from build123d import *

# Parameters (mm, degrees)
SKETCH_1_W                   = 80
SKETCH_1_H                   = 100
EXTRUDE_1_DEPTH              = 11
SKETCH_7_W                   = 15
SKETCH_7_H                   = 30
CUT_EXTRUDE_1_DEPTH          = 16
HOLE_WIZARD_M4_1_D           = 3.3
HOLE_WIZARD_M4_1_CSINK_D     = 4.05
HOLE_WIZARD_M4_1_CSINK_ANGLE = 90
FILLET_1_R                   = 20
FILLET_2_R                   = 2
SKETCH_9_W                   = 6
SKETCH_9_H                   = 35
CUT_EXTRUDE_2_DEPTH          = 11
SKETCH_11_R                  = 3
CUT_EXTRUDE_4_DEPTH          = 15
SKETCH_15_R                  = 1.9
CUT_EXTRUDE_8_DEPTH          = 14
SKETCH_16_R                  = 4.52
CUT_EXTRUDE_9_DEPTH          = 8.5
CUT_EXTRUDE_10_DEPTH         = 8.5
CUT_EXTRUDE_11_DEPTH         = 13.5
FILLET_4_R                   = 5
FILLET_5_R                   = 2


with BuildPart() as part:
    # 草图1 → 凸台-拉伸1 (new body)
    with BuildSketch(Plane.XY):
        Rectangle(SKETCH_1_W, SKETCH_1_H)
    extrude(amount=EXTRUDE_1_DEPTH)

    # 草图7 → 切除-拉伸1 (cut)
    with BuildSketch(Plane.XY.offset(11)):
        with Locations((0, 35)):
            Rectangle(SKETCH_7_W, SKETCH_7_H)
    extrude(amount=-CUT_EXTRUDE_1_DEPTH, mode=Mode.SUBTRACT)

    # M4 螺纹孔1 (through all)
    with Locations(Plane(origin=(13.5, 24.75, 0), x_dir=(-1, 0, 0), z_dir=(0, 0, -1))):
        with Locations((0, 0), (27, 0), (41.5, -49.5), (-14.5, -49.5)):
            CounterSinkHole(HOLE_WIZARD_M4_1_D / 2, HOLE_WIZARD_M4_1_CSINK_D / 2, counter_sink_angle=HOLE_WIZARD_M4_1_CSINK_ANGLE)

    # 圆角1
    fillet_1_edges = [part.edges().sort_by_distance(p)[0] for p in [
        (-40, 50, 5.5),
        (40, 50, 5.5),
    ]]
    fillet(fillet_1_edges, radius=FILLET_1_R)

    # 圆角2
    fillet_2_edges = [part.edges().sort_by_distance(p)[0] for p in [
        (-7.5, 20, 5.5),
        (-7.5, 50, 5.5),
        (7.5, 50, 5.5),
        (7.5, 20, 5.5),
        (40, -50, 5.5),
        (-40, -50, 5.5),
    ]]
    fillet(fillet_2_edges, radius=FILLET_2_R)

    # 草图9 → 切除-拉伸2 (cut)
    with BuildSketch(Plane.XY):
        with Locations((37, 0)):
            Rectangle(SKETCH_9_W, SKETCH_9_H)
        with Locations((-37, 0)):
            Rectangle(SKETCH_9_W, SKETCH_9_H)
    extrude(amount=CUT_EXTRUDE_2_DEPTH, mode=Mode.SUBTRACT)

    # 草图11 → 切除-拉伸4 (cut)
    with BuildSketch(Plane.XY):
        with Locations((-22.273863607, 38.273863607)):
            Circle(SKETCH_11_R)
        with Locations((22.273863607, 38.273863607)):
            Circle(SKETCH_11_R)
        with Locations((22.273863607, -6.273863607)):
            Circle(SKETCH_11_R)
        with Locations((-22.273863607, -6.273863607)):
            Circle(SKETCH_11_R)
    extrude(amount=CUT_EXTRUDE_4_DEPTH, mode=Mode.SUBTRACT)

    # 草图15 → 切除-拉伸8 (cut)
    with BuildSketch(Plane.XY.offset(11)):
        with Locations((-13.5, 24.75)):
            Circle(SKETCH_15_R)
        with Locations((-28, -24.75)):
            Circle(SKETCH_15_R)
        with Locations(Location((13.5, 24.75, 0), (0, 0, 180))):
            Circle(SKETCH_15_R)
        with Locations(Location((28, -24.75, 0), (0, 0, 180))):
            Circle(SKETCH_15_R)
    extrude(amount=-CUT_EXTRUDE_8_DEPTH, mode=Mode.SUBTRACT)

    # 草图16 → 切除-拉伸9 (cut)
    with BuildSketch(Plane(origin=(0, 0, 0), x_dir=(-1, 0, 0), z_dir=(0, 0, -1))):
        with Locations((-22.273863607, 38.273863607)):
            Circle(SKETCH_16_R)
        with Locations((-22.273863607, -6.273863607)):
            Circle(SKETCH_16_R)
        with Locations(Location((22.273863607, -6.273863607, 0), (0, 0, 180))):
            Circle(SKETCH_16_R)
        with Locations(Location((22.273863607, 38.273863607, 0), (0, 0, 180))):
            Circle(SKETCH_16_R)
    extrude(amount=-CUT_EXTRUDE_9_DEPTH, mode=Mode.SUBTRACT)

    # 草图17 → 切除-拉伸10 (cut)
    with BuildSketch(Plane.XY.offset(11)):
        Polygon((-15.468764418, 21.34), (-11.531235582, 21.34), (-9.562471164, 24.75), (-11.531235582, 28.16), (-15.468764418, 28.16), (-17.437528836, 24.75), align=None)
        Polygon((-26.031235582, -28.16), (-24.062471164, -24.75), (-26.031235582, -21.34), (-29.968764418, -21.34), (-31.937528836, -24.75), (-29.968764418, -28.16), align=None)
        Polygon((29.968764418, -28.16), (26.031235582, -28.16), (24.062471164, -24.75), (26.031235582, -21.34), (29.968764418, -21.34), (31.937528836, -24.75), align=None)
        Polygon((17.437528836, 24.75), (15.468764418, 21.34), (11.531235582, 21.34), (9.562471164, 24.75), (11.531235582, 28.16), (15.468764418, 28.16), align=None)
    extrude(amount=-CUT_EXTRUDE_10_DEPTH, mode=Mode.SUBTRACT)

    # 草图18 → 切除-拉伸11 (cut)
    with BuildSketch(Plane.XY.offset(11)):
        Polygon((-52.225177231, -29.5), (-20, -29.5), (-20, -24.5), (20, -24.5), (20, -29.5), (49.13660357, -29.5), (49.13660357, -55.082609568), (-52.225177231, -55.082609568), align=None)
    extrude(amount=-CUT_EXTRUDE_11_DEPTH, mode=Mode.SUBTRACT)

    # 圆角4
    fillet_4_edges = [part.edges().sort_by_distance(p)[0] for p in [
        (40, -29.5, 5.5),
        (-40, -29.5, 5.5),
    ]]
    fillet(fillet_4_edges, radius=FILLET_4_R)

    # 圆角5
    fillet_5_edges = [part.edges().sort_by_distance(p)[0] for p in [
        (-20, -27, 0),
        (-20, -29.5, 5.5),
        (0, -24.5, 0),
        (-20, -24.5, 5.5),
        (20, -27, 0),
        (20, -24.5, 5.5),
        (20, -29.5, 5.5),
        (20, -27, 11),
        (0, -24.5, 11),
        (-20, -27, 11),
    ]]
    fillet(fillet_5_edges, radius=FILLET_5_R)


solid = part.part
Check sheet for the modelled part. Datum: model origin and axes. Units: mm. A direction names the side the tool comes from. Give positions to 0.01 mm unless a question says otherwise; leave off trailing zeros. Write each loop counter-clockwise with the first axis right and the second up, starting at its lowest first coordinate (ties: lowest second). Pieces come first, ordered by that corner, then holes. Notation, with made-up numbers: (-4.5, -11) -> (2.5, -11) arc R25 ccw to (2.5, 19) -> close; hole circle Ø8 at (-22.75, -7). An arc over 180 degrees is marked (long way). Write item = value, one per line.
Item 1: Tool access check on faces 1 (the flat face through (30.967, -26.431, 6.81)), 2 (the flat face through (7.5, 35, 6)), 3 (the flat face through (34, 0, 5)), 4 (the flat face through (0, -24.5, 6)). Record the directions out of +Z, -Z, +X, -X, +Y, -Y that give a thin tool (end or side, any length) a straight path to the whole face; none if there is none.
Output:
face_1 = +Z
face_2 = +Z, -Z, +Y
face_3 = +Z, -Z, +X
face_4 = +Z, -Z, -Y
Item 2: Sectioned sample at B-B on x = 4. Record the boundary of the cut face in (y, z).
Output:
outline = (-24.5, 2) arc R2 ccw to (-22.5, 0) -> (20, 0) -> (20, 11) -> (-22.5, 11) arc R2 ccw to (-24.5, 9) -> close
Item 3: Sectioned sample at A-A on x = -13.5. Record the boundary of the cut face in (y, z) (3 decimals).
Output:
outline = (-24.5, 2) arc R2 ccw to (-22.5, 0) -> (22.725, 0) -> (22.85, 0.125) -> (22.85, 2.5) -> (21.34, 2.5) -> (21.34, 11) -> (-22.5, 11) arc R2 ccw to (-24.5, 9) -> close; (26.65, 0.125) -> (26.775, 0) -> (50, 0) -> (50, 11) -> (28.16, 11) -> (28.16, 2.5) -> (26.65, 2.5) -> close
Item 4: Gauge pin test, flat ends, axial feed: pin 1 (5.5 mm diameter, centred on y = -1, z = 3.5, fed in from +X); pin 2 (1 mm diameter, centred on y = 38, z = 1.5, fed in from -X); pin 3 (2 mm diameter, centred on x = -27.5, y = -24.5, fed in from +Z); pin 4 (5 mm diameter, centred on x = -7.5, z = 5, fed in from -Y). Record the tip position at first contact, or that the pin passes through.
Output:
pin_1 = 34
pin_2 = -38.54
pin_3 = through
pin_4 = -24.5
Item 5: Release check for a two-part mould opening along X. For faces 5 (the cylindrical face through (33.986, 44.297, 5.577)), 6 (the flat face through (-10.533, 26.431, 6.81)), 7 (the cylindrical face through (-38.57, -28, 5.58)) record: +X half, -X half, draft (parallel to the pull), parting line (faces both ways), or undercut.
Output:
face_5 = +X half
face_6 = undercut
face_7 = -X half
Item 6: Sectioned sample at C-C on x = -28. Record the boundary of the cut face in (y, z) (3 decimals), and give its area (3 significant figures).
Output:
outline = (-29.5, 0) -> (-26.775, 0) -> (-26.65, 0.125) -> (-26.65, 2.5) -> (-28.16, 2.5) -> (-28.16, 11) -> (-29.5, 11) -> close; (-22.85, 0.125) -> (-22.725, 0) -> (48.33, 0) -> (48.33, 11) -> (-21.34, 11) -> (-21.34, 2.5) -> (-22.85, 2.5) -> close
area = 789 mm^2
Item 7: Scan lines: probe 1 along Y at (x, z) = (12.5, 6); probe 2 along Y at (x, z) = (-19, 4.25); probe 3 along Y at (x, z) = (-13.5, 1.75). Record each from-to range of solid material in increasing order. Write a range as from..to.
Output:
probe_1 = -24.5..21.34, 28.16..50
probe_2 = -24.77..-9.39, -3.16..35.16, 41.39..50
probe_3 = -24.48..22.85, 26.65..50
Item 8: Sectioned sample at D-D on z = 4.75. Count the separate pieces of the cut face and the enclosed holes in it, and give its area (3 significant figures).
Output:
separate_pieces = 1
enclosed_holes = 8
area = 4,690 mm^2
